The drawing under review shows one solid part. Ordinate dimensions are in mm from its lowest x, y, z. A direction names the side the tool comes from. Give positions to 0.01 mm unless a question says otherwise; leave off trailing zeros. Write each loop counter-clockwise with the first axis right and the second up, starting at its lowest first coordinate (ties: lowest second). Pieces come first, ordered by that corner, then holes. Notation, with made-up numbers: (45, 49) - (96, 49) arc R15 ccw to (96, 78) - close; hole circle Ø6 at (23, -36.5). An arc over 180 degrees is marked (long way). Write item = value, one per line.
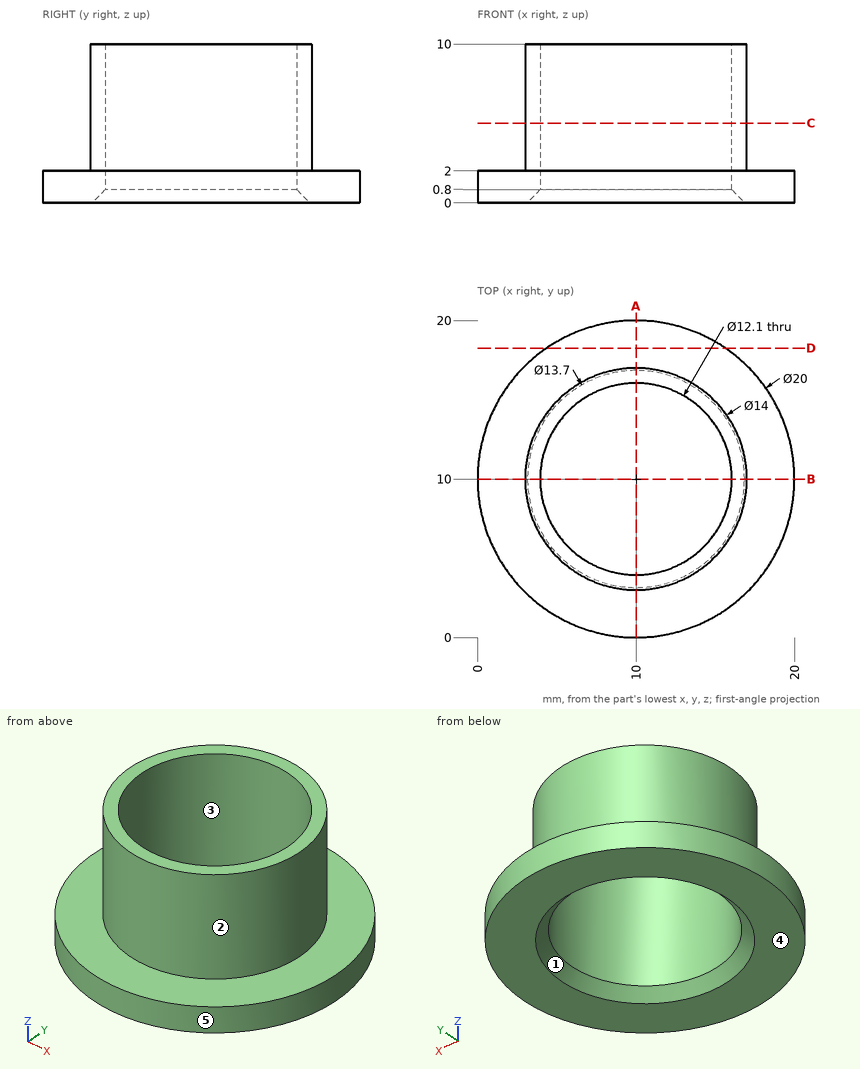
1. Insertion check: P1, Ø1.5, axis at x = 15, y = 4.5, coming from the +Z side; P2, Ø1, axis at y = 14.5, z = 5.5, coming from the +X side; P3, Ø3, axis at x = 2.5, y = 16.5, coming from the +Z side. Each pin has a flat end and moves straight along its axis. Give the tip position at first contact, or say it passes through.
Findings below:
P1 = 10
P2 = 15.74
P3 = 2
2. Take a section at C-C on z = 5. Give the boundary of the cut face in (x, y), and give its area (3 significant figures).
Findings below:
outline = circle Ø14 at (10, 10); hole circle Ø12.1 at (10, 10)
area = 38.9 mm²
3. Take a section at A-A on x = 10. Give the boundary of the cut face in (y, z).
Findings below:
outline = (0, 0) - (3.15, 0) - (3.95, 0.8) - (3.95, 10) - (3, 10) - (3, 2) - (0, 2) - close; (16.05, 0.8) - (16.85, 0) - (20, 0) - (20, 2) - (17, 2) - (17, 10) - (16.05, 10) - close
4. Take a section at D-D on y = 18.25. Give the boundary of the cut face in (x, z), and give its area (3 significant figures).
Findings below:
outline = (4.35, 0) - (15.65, 0) - (15.65, 2) - (4.35, 2) - close
area = 22.6 mm²
5. Draft analysis for pull direction X (two halves, no side actions). For the marked faces 3, 4 and 5, state which applies: +X half, -X half, draft (parallel to the pull), parting line (faces both ways), or undercut.
Findings below:
face_3 = undercut
face_4 = draft
face_5 = parting line
6. For line 1 (Y direction, x = 10, z = 5.25); line 2 (Z direction, x = 17.5, y = 4.25); line 3 (X direction, y = 9.25, z = 1.5), list the stretches that pass through material, from the lowest coordinate up. Write a range as from..to.
Findings below:
line_1 = 3..3.95, 16.05..17
line_2 = 0..2
line_3 = 0.03..4, 16..19.97
7. Machinability: for the marked faces 1 and 2, which of the approach directions +Z, -Z, +X, -X, +Y, -Y give a long, thin tool a straight path to every point of the face, cutting with its end or side? Answer none if there is none.
Findings below:
face_1 = -Z
face_2 = +Z
